Autodesk Inventor part; units mm, degrees
ref_plane "YZ Plane" through (0, 0, 0) normal (1, 0, 0) x (0, 1, 0)
ref_plane "XZ Plane" through (0, 0, 0) normal (0, 1, 0) x (-1, 0, 0)
ref_plane "XY Plane" through (0, 0, 0) normal (0, 0, 1) x (1, 0, 0)
sketch "Sketch2" plane through (0, 0, 0) normal (0, 0, 1) x (1, 0, 0)
  line L0 (-17, 28) -> (0, 28)
  line L1 (0, 28) -> (0, 17)
  line L2 (0, 7) -> (0, 0)
  line L3 (0, 0) -> (-17, 0)
  line L4 (-17, 0) -> (-17, 7)
  line L5 (-17, 28) -> (-17, 17)
  line L6 (-17, 17) -> (-17, 7)
  line L7 (0, 17) -> (0, 7)
  dimension "d0" = 17
  dimension "d1" = 28
extrude "Extrusion1" add sketch "Sketch2" along normal blind 5
sketch "Sketch4" plane through (0, 0, 0) normal (0, 0, -1) x (-1, 0, 0)
  line L0 (17, 28) -> (0, 28)
  line L1 (0, 28) -> (0, 0)
  line L2 (0, 0) -> (17, 0)
  line L3 (17, 0) -> (17, 28)
  line L4 (0, 28) -> (17, 28)
  line L5 (11.5, 24) -> (11.5, 4)
  line L6 (11.5, 4) -> (5.5, 4)
  line L7 (5.5, 4) -> (5.5, 24)
  line L8 (5.5, 24) -> (11.5, 24)
  dimension "d15" = 6
  dimension "d17" = 5.5
  dimension "d30" = 20
  dimension "d31" = 4
extrude "Extrusion3" cut sketch "Sketch4" against normal blind 1.5 contours L5 L6 L7 L8
sketch "Sketch5" plane through (0, 0, 5) normal (0, 0, 1) x (1, 0, 0)
  line L0 (0, 28) -> (-17, 28)
  line L1 (-17, 28) -> (-17, 0)
  line L2 (-17, 0) -> (0, 0)
  line L3 (0, 0) -> (0, 28)
  line L4 (-21, 17) -> (4, 7)
  line L5 (-21.4753, 7) -> (4, 17)
  circle A0 centre (-8.6177, 12.0471) radius 5
  dimension "d20" = 10
  dimension "d21" = 12.0471
extrude "Extrusion4" cut sketch "Sketch5" against normal through all contours A0 L4 L5 | L5 L4 A0 | L4 L5 A0 | A0 L5 L4
sketch "Sketch6" plane through (0, 0, 5) normal (0, 0, 1) x (1, 0, 0)
  circle A0 centre (-8.6177, 12.0471) radius 5
  line L0 (0, 28) -> (-17, 28)
  line L1 (-17, 28) -> (-17, 0)
  line L2 (-17, 0) -> (0, 0)
  line L3 (0, 0) -> (0, 28)
  circle A1 centre (-12.5, 26) radius 1.35
  dimension "d24" = 2.7
  dimension "d25" = 4.5
  dimension "d26" = 2
extrude "Extrusion5" cut sketch "Sketch6" against normal through all contours A1
sketch "Sketch7" plane through (0, 0, 5) normal (0, 0, 1) x (1, 0, 0)
  line L0 (0, 0) -> (0, 28)
  line L1 (-17, 0) -> (0, 0)
  circle A0 centre (-4.5, 5) radius 1.35
  point P0 (0, 7)
  dimension "d32" = 2.7
  dimension "d33" = 4.5
  dimension "d34" = 5
extrude "Extrusion6" cut sketch "Sketch7" against normal through all
sketch "Sketch8" plane through (0, 0, 0) normal (1, 0, 0) x (0, 0, -1)
  circle A0 centre (-2.5, 12.5) radius 1.6
  line L0 (-5, 0) -> (-5, 28)
  line L1 (0, 0) -> (-5, 0)
  point P0 (0, -7)
  dimension "d37" = 3.2
  dimension "d41" = 12.5
  dimension "d49" = 2.5
extrude "Extrusion8" cut sketch "Sketch8" against normal through all
sketch "Sketch9" plane through (0, 0, 5) normal (0, 0, 1) x (1, 0, 0)
  circle A0 centre (-4.5, 5) radius 1.35
  circle A1 centre (-12.5, 26) radius 1.35
  circle A2 centre (-8.6177, 12.0471) radius 5
  line L0 (0, 28) -> (-17, 28)
  line L1 (-17, 28) -> (-17, 0)
  line L2 (-17, 0) -> (0, 0)
  line L3 (0, 0) -> (0, 28)
  line L4 (-17, 0) -> (-16.5, 0)
  line L5 (-16.5, 0) -> (-16.5, 28)
  line L6 (-16.5, 28) -> (-17, 28)
  line L7 (-17, 28) -> (-17, 0)
  line L8 (0, 0) -> (-0.5, 0)
  line L9 (-0.5, 0) -> (-0.5, 28)
  line L10 (-0.5, 28) -> (0, 28)
  line L11 (0, 28) -> (0, 0)
  dimension "d47" = 0.5
  dimension "d48" = 0.5
extrude "Extrusion9" cut sketch "Sketch9" against normal through all contours L3 L2 L9 L0 | L5 L2 L1 L0
properties part number "tapaB0.2"
For this review, take the finished solid that the model builds, in its own axes (mm). A direction names the side the tool comes from. Round coordinates to 2 decimals unless told otherwise and drop trailing zeros. Loops run counter-clockwise (first coordinate to the right, second up) from the corner with the lowest first, then second, coordinate; pieces in that order, holes last. Notation, with made-up numbers: (23, 86) - (48, 86) arc R28 cw to (48, 104) - close; hole circle Ø4 at (55.25, 86.25). An arc over 180 degrees is marked (long way). Use one line per item in the form item = value.
Item 1: Clearance check with a flat-ended pin moving along its axis: P1, Ø1.2, axis at x = -9.5, y = 5.5, coming from the -Z side. State where the tip first meets the part, or that it passes through.
Answers:
P1 = 1.5
Item 2: Consider section A-A on y = 26. Write out the cut boundary in (x, z).
Answers:
outline = (-16.5, 0) - (-13.85, 0) - (-13.85, 5) - (-16.5, 5) - close; (-11.15, 0) - (-0.5, 0) - (-0.5, 5) - (-11.15, 5) - close
Item 3: Mouldability with a two-part tool opening along X and no side actions: class faces 3 (the flat face through (-0.5, 14, 4)), 4 (the cylindrical face through (-2.254, 14.086, 2.708)), 5 (the flat face through (-16.5, 14, 4)), 6 (the flat face through (-11.5, 20, 1)) as +X half, -X half, draft (parallel to the pull), parting line (faces both ways), or undercut.
Answers:
face_3 = +X half
face_4 = draft
face_5 = -X half
face_6 = undercut
Item 4: Consider section D-D on x = -12.5. Write out the cut boundary in (y, z).
Answers:
outline = (0, 0) - (8.9, 0) - (8.9, 5) - (0, 5) - close; (15.2, 0) - (24.65, 0) - (24.65, 5) - (15.2, 5) - close; (27.35, 0) - (28, 0) - (28, 5) - (27.35, 5) - close
Item 5: Tool access review of faces 1 (the flat face through (-8.6, 17.3, 5)), 2 (the flat face through (-5.5, 20, 1)): name each direction out of +Z, -Z, +X, -X, +Y, -Y from which nothing blocks a thin tool from reaching the whole face with its end or side.
Answers:
face_1 = +Z, +X, -X, +Y, -Y
face_2 = -Z
Item 6: Consider section B-B on z = 2.5. Write out the cut boundary in (x, y).
Answers:
outline = (-16.5, 0) - (-0.5, 0) - (-0.5, 10.9) - (-3.75, 10.9) arc R5 cw to (-13.48, 10.9) - (-16.5, 10.9) - close; (-16.5, 14.1) - (-13.18, 14.1) arc R5 cw to (-4.06, 14.1) - (-0.5, 14.1) - (-0.5, 28) - (-16.5, 28) - close; hole circle Ø2.7 at (-12.5, 26); hole circle Ø2.7 at (-4.5, 5)
Item 7: Consider section C-C on x = -8.5. Write out the cut boundary in (y, z).
Answers:
outline = (0, 0) - (4, 0) - (4, 1.5) - (7.05, 1.5) - (7.05, 5) - (0, 5) - close; (17.05, 1.5) - (24, 1.5) - (24, 0) - (28, 0) - (28, 5) - (17.05, 5) - close
Item 8: For line 1 (Y direction, x = -8.25, z = 0.6); line 2 (Y direction, x = -12, z = 2); line 3 (Y direction, x = -2.1, z = 2.5), list the stretches that pass through material, from the lowest coordinate up.
Answers:
line_1 = 0 to 4, 24 to 28
line_2 = 0 to 8.36, 15.73 to 24.75, 27.25 to 28
line_3 = 0 to 10.9, 14.1 to 28
